from build123d import *

# Parameters (mm, degrees)
ESQUISSE1_R             = 6
BOSS_EXTRU_1_DEPTH      = 8
ESQUISSE2_W             = 29
ESQUISSE2_H             = 18
BOSS_EXTRU_2_DEPTH      = 4
ESQUISSE3_W             = 29
ESQUISSE3_H             = 18
ESQUISSE3_W_2           = 23
ESQUISSE3_H_2           = 12
BOSS_EXTRU_3_DEPTH      = 4
ENL_V_MAT_EXTRU_1_DEPTH = 4


with BuildPart() as part:
    # Esquisse1 → Boss.-Extru.1 (new body)
    with BuildSketch(Plane(origin=(0, 0, 0), x_dir=(1, 0, 0), z_dir=(0, 1, 0))):
        with BuildLine():
            Line((0, 0), (6, 0))
            Line((6, 0), (36, 0))
            Line((36, 0), (62, 0))
            Line((62, 0), (62, 28.055987731))
            Line((62, 28.055987731), (36, 28.055987731))
            ThreePointArc((36, 28.055987731), (9.034681758, 34.39083629), (6, 61.923533231))
            Line((6, 61.923533231), (6, 62.923533231))
            ThreePointArc((6, 62.923533231), (4.535533906, 66.459067137), (1, 67.923533231))
            Line((1, 67.923533231), (0, 67.923533231))
            Line((0, 67.923533231), (0, 0))
        make_face()
        with Locations((51, 12.304583192)):
            Circle(ESQUISSE1_R, mode=Mode.SUBTRACT)
    extrude(amount=BOSS_EXTRU_1_DEPTH)

    # Esquisse2 → Boss.-Extru.2 (add)
    with BuildSketch(Plane(origin=(0, 8, 0), x_dir=(1, 0, 0), z_dir=(0, 1, 0))):
        with Locations((45.5, 12.304583192)):
            Rectangle(ESQUISSE2_W, ESQUISSE2_H)
        with BuildLine():
            Line((45, 15.304583192), (45.255437353, 15.304583192))
            ThreePointArc((45.255437353, 15.304583192), (45.718347403, 15.418177932), (46.07608916, 15.733154621))
            ThreePointArc((46.07608916, 15.733154621), (57, 12.304583192), (46.07608916, 8.876011764))
            ThreePointArc((46.07608916, 8.876011764), (45.718347403, 9.190988453), (45.255437353, 9.304583192))
            Line((45.255437353, 9.304583192), (45, 9.304583192))
            ThreePointArc((45, 9.304583192), (42, 12.304583192), (45, 15.304583192))
        make_face(mode=Mode.SUBTRACT)
    extrude(amount=BOSS_EXTRU_2_DEPTH)

    # Esquisse3 → Boss.-Extru.3 (add)
    with BuildSketch(Plane(origin=(0, 12, 0), x_dir=(1, 0, 0), z_dir=(0, 1, 0))):
        with Locations((45.5, 12.304583192)):
            Rectangle(ESQUISSE3_W, ESQUISSE3_H)
        with Locations((45.5, 12.304583192)):
            Rectangle(ESQUISSE3_W_2, ESQUISSE3_H_2, mode=Mode.SUBTRACT)
    extrude(amount=BOSS_EXTRU_3_DEPTH)

    # Esquisse4 → Enlèv. mat.-Extru.1 (cut)
    with BuildSketch(Plane.XZ):
        Polygon((47.7, -17.055987731), (54.3, -17.055987731), (55.193703609, -16.162284122), (57.721788353, -28.055987731), (54.3, -28.055987731), (47.7, -28.055987731), (44.278211647, -28.055987731), (46.806296391, -16.162284122), align=None)
    extrude(amount=-ENL_V_MAT_EXTRU_1_DEPTH, mode=Mode.SUBTRACT)


solid = part.part
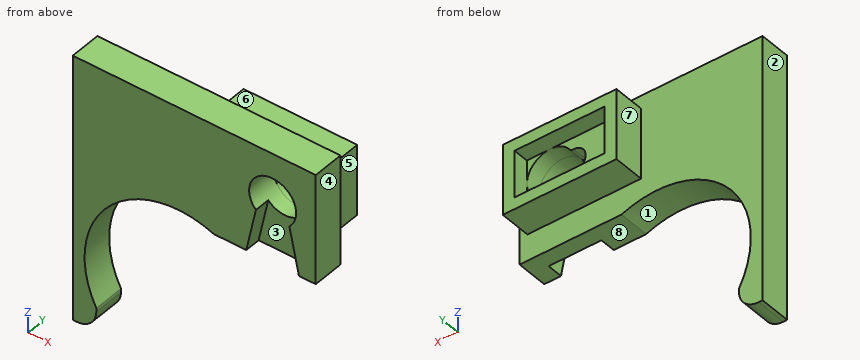
For this review, take the finished solid that the model builds, in its own axes (mm). Face numbers are marked on the shaded views. A direction names the side the tool comes from. Round coordinates to 2 decimals unless told otherwise and drop trailing zeros. Loops run counter-clockwise (first coordinate to the right, second up) from the corner with the lowest first, then second, coordinate; pieces in that order, holes last. Notation, with made-up numbers: (58, -29.75) - (112, -29.75) arc R13 cw to (112, -18.75) - close; hole circle Ø5 at (40.5, 85). An arc over 180 degrees is marked (long way). Use one line per item in the form item = value.
Item 1: Consider section A-A on y = 14.5. Write out the cut boundary in (x, z), then the cut area to 3 significant figures.
Answers:
outline = (31, -21.3) - (60, -21.3) - (60, -3.3) - (31, -3.3) - close; hole (34, -18.3) - (57, -18.3) - (57, -6.3) - (34, -6.3) - close
area = 246 mm^2
Item 2: Clearance check with flat-ended pins moving along their axes: P1, Ø1.1, axis at y = 4, z = -62, coming from the +X side; P2, Ø6, axis at x = 49.5, z = -21.5, coming from the -Y side; P3, Ø2, axis at x = 43, z = -11.5, coming from the +Y side. State where each tip first meets the part, or that it passes through.
Answers:
P1 = 6
P2 = 4
P3 = 12
Item 3: Tool access review of the marked faces 5, 6, 7 and 8: name each direction out of +Z, -Z, +X, -X, +Y, -Y from which nothing blocks a thin tool from reaching the whole face with its end or side.
Answers:
face_5 = +Z, -Z, +X, +Y
face_6 = +Z, +X, -X, +Y
face_7 = +Z, -Z, -X, +Y
face_8 = -Z, +X, +Y, -Y
Item 4: For line 1 (X direction, y = 12.5, z = -17.5); line 2 (Z direction, x = 51, y = 4.75); line 3 (Z direction, x = 54, y = 4.75), list the stretches that pass through material, from the lowest coordinate up.
Answers:
line_1 = 31 to 34, 57 to 60
line_2 = -28.06 to -18.3, -6.3 to 0
line_3 = -28.06 to -17.5, -7.11 to 0
Item 5: Consider section B-B on z = -8. Write out the cut boundary in (x, y).
Answers:
outline = (0, 0) - (46.82, 0) - (46.82, 12) - (34, 12) - (34, 16) - (31, 16) - (31, 8) - (0, 8) - close; (55.18, 0) - (62, 0) - (62, 8) - (60, 8) - (60, 16) - (57, 16) - (57, 12) - (55.18, 12) - close
Item 6: Mouldability with a two-part tool opening along X and no side actions: class the marked faces 1, 2, 3 and 4 as +X half, -X half, draft (parallel to the pull), parting line (faces both ways), or undercut.
Answers:
face_1 = undercut
face_2 = -X half
face_3 = undercut
face_4 = +X half
Item 7: Consider section C-C on y = 2. Write out the cut boundary in (x, z).
Answers:
outline = (0, -67.92) - (1, -67.92) arc R5 ccw to (6, -62.92) - (6, -61.92) arc R24 cw to (36, -28.06) - (44.28, -28.06) - (46.73, -16.52) arc R6 cw (long way) to (55.27, -16.52) - (57.72, -28.06) - (62, -28.06) - (62, 0) - (0, 0) - close
Item 8: Consider section D-D on x = 48. Write out the cut boundary in (y, z), then the cut area to 3 significant figures.
Answers:
outline = (0, -7.11) - (12, -7.11) - (12, -6.3) - (16, -6.3) - (16, -3.3) - (8, -3.3) - (8, 0) - (0, 0) - close; (4, -28.06) - (8, -28.06) - (8, -21.3) - (16, -21.3) - (16, -18.3) - (12, -18.3) - (12, -17.5) - (4, -17.5) - close
area = 154 mm^2
